Geometry: final body of the model. Coordinates: model frame, mm. A direction names the side the tool comes from. Round coordinates to 2 decimals unless told otherwise and drop trailing zeros. Order: outer loops, then holes, each group sorted by start corner. A loop starts at its lowest first (then second) coordinate and runs counter-clockwise, first axis right, second up. Notation, with made-up numbers: (-8, -4) - (11, -4) arc R23 ccw to (11, 12) - close; hole circle Ø8 at (52.25, -24.75). An arc over 180 degrees is marked (long way). Put each result on its own line as item: value. Start each with the question number.
(1) Material intervals for L1, parallel to X at y = -4, z = -28; L2, parallel to Y at x = 7, z = -12 (3 decimals); L3, parallel to X at y = 3, z = -4.5 (3 decimals), sorted ascending. Write a range as [from, to].
(2) Section B-B (x = -5). Output: boundary loops of the cut face in (y, z) (3 decimals).
(3) Pin query (flat end, axial travel): P1, Ø2, axis at x = 7, y = 22, coming from the -Z side; P2, Ø1.6, axis at x = 7, y = 44, coming from the -Z side. Return the tip coordinate at first contact, or that it passes through.
(4) Pull-direction query (X, two-part tool) for faces 4 (the face through (-12.5, 20, -16)), 5 (the face through (0, -10, -16)), 6 (the face through (8.183, 44.658, -26.077)); classes: released by +X, released by -X, zero draft, split by the parting line, or undercut.
(5) Section D-D (z = -26). Output: boundary loops of the cut face in (x, y) (3 decimals), and give its area (3 significant figures).
(6) Section C-C (z = -10.5). Output: boundary loops of the cut face in (x, y) (3 decimals).
(7) Access query for faces 1 (the face through (12.5, 20, -16)), 2 (the face through (3, 48, -18)), 3 (the face through (4, 42, -15)). Directions: +Z, -Z, +X, -X, +Y, -Y. A direction counts if a zero-diameter tool reaches every point of the face in a straight line with its end or side. Return the directions, or none.
(8) Section A-A (y = 44). Output: boundary loops of the cut face in (x, z), and give its area (3 significant figures).
from build123d import *

# Parameters (mm, degrees)
SKETCH1_W           = 31.5
SKETCH1_H           = 60
BOSS_EXTRUDE1_DEPTH = 12.5
SKETCH2_W           = 5.015
SKETCH2_H           = 40.03
SKETCH2_W_2         = 8
SKETCH2_H_2         = 3.985
CUT_EXTRUDE1_DEPTH  = 27.53
SKETCH6_R           = 3.25
CUT_EXTRUDE2_DEPTH  = 11


with BuildPart() as part:
    # Sketch1 → Boss-Extrude1 (new, symmetric)
    with BuildSketch(Plane(origin=(0, 0, 0), x_dir=(0, 0, -1), z_dir=(1, 0, 0))):
        with Locations((15.75, 20)):
            Rectangle(SKETCH1_W, SKETCH1_H)
    extrude(amount=BOSS_EXTRUDE1_DEPTH, both=True)

    # Sketch2 → Cut-Extrude1 (cut)
    with BuildSketch(Plane(origin=(0, 0, -31.5), x_dir=(-1, 0, 0), z_dir=(0, 0, -1))):
        with Locations((-7.5075, 20)):
            Rectangle(SKETCH2_W, SKETCH2_H)
        Polygon((-5, -0.015), (5, -0.015), (5, 40.015), (4, 40.015), (-4, 40.015), (-5, 40.015), align=None)
        with Locations((7.5075, 20)):
            Rectangle(SKETCH2_W, SKETCH2_H)
        with Locations((0, 42.0075)):
            Rectangle(SKETCH2_W_2, SKETCH2_H_2)
        Polygon((-4, 44), (4, 44), (4, 45), (3, 45), (3, 50), (-3, 50), (-3, 45), (-4, 45), align=None)
    extrude(amount=-CUT_EXTRUDE1_DEPTH, mode=Mode.SUBTRACT)

    # Sketch6 → Cut-Extrude2 (cut)
    with BuildSketch(Plane(origin=(0, 0, -31.5), x_dir=(-1, 0, 0), z_dir=(0, 0, -1))):
        with Locations((-5, 44)):
            Circle(SKETCH6_R)
        with Locations((5, 44)):
            Circle(SKETCH6_R)
        with Locations(Location((5, -4, 0), (0, 0, 90))):
            Circle(SKETCH6_R)
        with Locations(Location((-5, -4, 0), (0, 0, 90))):
            Circle(SKETCH6_R)
    extrude(amount=-CUT_EXTRUDE2_DEPTH, mode=Mode.SUBTRACT)


solid = part.part
Checks:
1. L1: x = [-12.5, -8.25], [-1.75, 1.75], [8.25, 12.5]
1. L2: y = [-10, -0.015], [40.015, 50]
1. L3: x = [-12.5, -10.015], [10.015, 12.5]
2. outline: (-10, -31.5) - (-7.25, -31.5) - (-7.25, -20.5) - (-0.75, -20.5) - (-0.75, -31.5) - (-0.015, -31.5) - (-0.015, -3.97) - (40.015, -3.97) - (40.015, -31.5) - (40.75, -31.5) - (40.75, -20.5) - (47.25, -20.5) - (47.25, -31.5) - (50, -31.5) - (50, 0) - (-10, 0) - close
3. P1: stops at z = -3.97
3. P2: stops at z = -20.5
4. face 4: released by -X
4. face 5: zero draft
4. face 6: undercut
5. outline: (-12.5, -10) - (12.5, -10) - (12.5, 50) - (3, 50) - (3, 46.562) arc R3.25 cw (long way) to (4, 40.908) - (4, 40.015) - (10.015, 40.015) - (10.015, -0.015) - (-10.015, -0.015) - (-10.015, 40.015) - (-4, 40.015) - (-4, 40.908) arc R3.25 cw (long way) to (-3, 46.562) - (-3, 50) - (-12.5, 50) - close; hole circle Ø6.5 at (-5, -4); hole circle Ø6.5 at (5, -4)
5. area: 512 mm²
6. outline: (-12.5, -10) - (12.5, -10) - (12.5, 50) - (3, 50) - (3, 45) - (4, 45) - (4, 40.015) - (10.015, 40.015) - (10.015, -0.015) - (-10.015, -0.015) - (-10.015, 40.015) - (-4, 40.015) - (-4, 45) - (-3, 45) - (-3, 50) - (-12.5, 50) - close
7. face 1: +Z, -Z, +X, +Y, -Y
7. face 2: -Z, +Y
7. face 3: -Z
8. outline: (-12.5, -31.5) - (-8.25, -31.5) - (-8.25, -20.5) - (-4, -20.5) - (-4, -3.97) - (4, -3.97) - (4, -20.5) - (8.25, -20.5) - (8.25, -31.5) - (12.5, -31.5) - (12.5, 0) - (-12.5, 0) - close
8. area: 474 mm²
